```python
from build123d import *

# Parameters (mm, degrees)
EXTRUDE_26_DEPTH       = 26
SKETCH_18_5_Y138_5_W   = 5
SKETCH_18_5_Y138_5_H   = 18
CUT_EXTRUDE_18_5_DEPTH = 1.2
FILLET_R0_5_R          = 0.5
FILLET_R0_5_2_R        = 0.5


with BuildPart() as part:
    # 草图_L形卡耳_内伸12_厚1点2_内R1点2_焊脚12 → 拉伸_卡耳外高26 (new body)
    with BuildSketch(Plane(origin=(0, 125.5, 0), x_dir=(1, 0, 0), z_dir=(0, 1, 0))):
        with BuildLine():
            Line((59.2, 303.8), (68.8, 303.8))
            ThreePointArc((68.8, 303.8), (70.497056275, 303.097056275), (71.2, 301.4))
            Line((71.2, 301.4), (71.2, 289.4))
            Line((71.2, 289.4), (70, 289.4))
            Line((70, 289.4), (70, 301.4))
            ThreePointArc((70, 301.4), (69.648528137, 302.248528137), (68.8, 302.6))
            Line((68.8, 302.6), (59.2, 302.6))
            Line((59.2, 302.6), (59.2, 303.8))
        make_face()
    extrude(amount=EXTRUDE_26_DEPTH)

    # 草图_卡槽矩形_净高18_净宽5_中心Y138点5 → 切除_卡槽18乘5 (cut)
    with BuildSketch(Plane.XY.offset(-302.6)):
        with Locations((65.5, 138.5)):
            Rectangle(SKETCH_18_5_Y138_5_W, SKETCH_18_5_Y138_5_H)
    extrude(amount=-CUT_EXTRUDE_18_5_DEPTH, mode=Mode.SUBTRACT)

    # Fillet R0_5
    fillet_r0_5_edges = [part.edges().sort_by_distance(p)[0] for p in [
        (68, 147.5, -303.2),
        (68, 129.5, -303.2),
        (63, 129.5, -303.2),
        (63, 147.5, -303.2),
    ]]
    fillet(fillet_r0_5_edges, radius=FILLET_R0_5_R)

    # Fillet R0_5 2
    fillet_r0_5_2_edges = [part.edges().sort_by_distance(p)[0] for p in [
        (59.2, 125.5, -303.2),
        (59.2, 151.5, -303.2),
    ]]
    fillet(fillet_r0_5_2_edges, radius=FILLET_R0_5_2_R)


solid = part.part
```
Input: part model. Units: mm. Frame: model coordinates. A direction names the side the tool comes from. Coordinates: 2 decimals unless noted, no trailing zeros. Write each loop counter-clockwise with the first axis right and the second up, starting at its lowest first coordinate (ties: lowest second). Pieces come first, ordered by that corner, then holes.
1) Pin query (flat end, axial travel): pin 1 Ø4 at (x, y) = (65.5, 129) entering from +Z; pin 2 Ø0.6 at (y, z) = (141.5, -303) entering from +X; pin 3 Ø5 at (y, z) = (139.5, -294.5) entering from -X. Return the tip coordinate at first contact, or that it passes through.
2) Mould query, pull axis X, two halves, no side actions, for faces 1 (the flat face through (62, 138, -302.6)), 2 (the cylindrical face through (70.478, 138.318, -303.116)), 3 (the flat face through (65, 147.5, -303)), 4 (the flat face through (70, 138, -295)). Classes: pulls with the +X half, pulls with the -X half, needs draft (parallel to the pull), parting line crosses it, or undercut.
3) Section D-D on x = 61.5. Output: boundary loops of the cut face in (y, z), and give its area (3 significant figures).
4) Section B-B on x = 64. Output: boundary loops of the cut face in (y, z).
5) Material intervals for line 1 along X through (y, z) = (136, -297.25); line 2 along Z through (x, y) = (68.5, 134); line 3 along Z through (x, y) = (70.25, 135.25), sorted ascending.
6) Section C-C on z = -294.5. Output: boundary loops of the cut face in (x, y), and give its area (3 significant figures).
7) Section A-A on y = 133.75. Output: boundary loops of the cut face in (x, z), and give its area (3 significant figures).
8) Set-up query: faces 5 (the flat face through (65, 129.5, -303)), 6 (the cylindrical face through (69.658, 138.318, -302.239)). Return all of +Z, -Z, +X, -X, +Y, -Y with unobstructed straight access to the full face (end or side cutting, diameter ignored); none if empty.
Check result:
1. pin 1: stops at z = -302.6
1. pin 2: stops at x = 70.82
1. pin 3: stops at x = 70
2. face 1: needs draft
2. face 2: pulls with the +X half
2. face 3: undercut
2. face 4: pulls with the -X half
3. outline: (125.5, -303.8) - (151.5, -303.8) - (151.5, -302.6) - (125.5, -302.6) - close
3. area: 31.2 mm2
4. outline: (125.5, -303.8) - (129.5, -303.8) - (129.5, -302.6) - (125.5, -302.6) - close; (147.5, -303.8) - (151.5, -303.8) - (151.5, -302.6) - (147.5, -302.6) - close
5. line 1: x = 70 to 71.2
5. line 2: z = -303.8 to -302.6
5. line 3: z = -303.31 to -289.4
6. outline: (70, 125.5) - (71.2, 125.5) - (71.2, 151.5) - (70, 151.5) - close
6. area: 31.2 mm2
7. outline: (59.2, -303.8) - (63, -303.8) - (63, -302.6) - (59.2, -302.6) - close; (68, -303.8) - (68.8, -303.8) arc R2.4 ccw to (71.2, -301.4) - (71.2, -289.4) - (70, -289.4) - (70, -301.4) arc R1.2 cw to (68.8, -302.6) - (68, -302.6) - close
7. area: 23.3 mm2
8. face 5: +Z, -Z
8. face 6: +Z, -X, +Y, -Y
